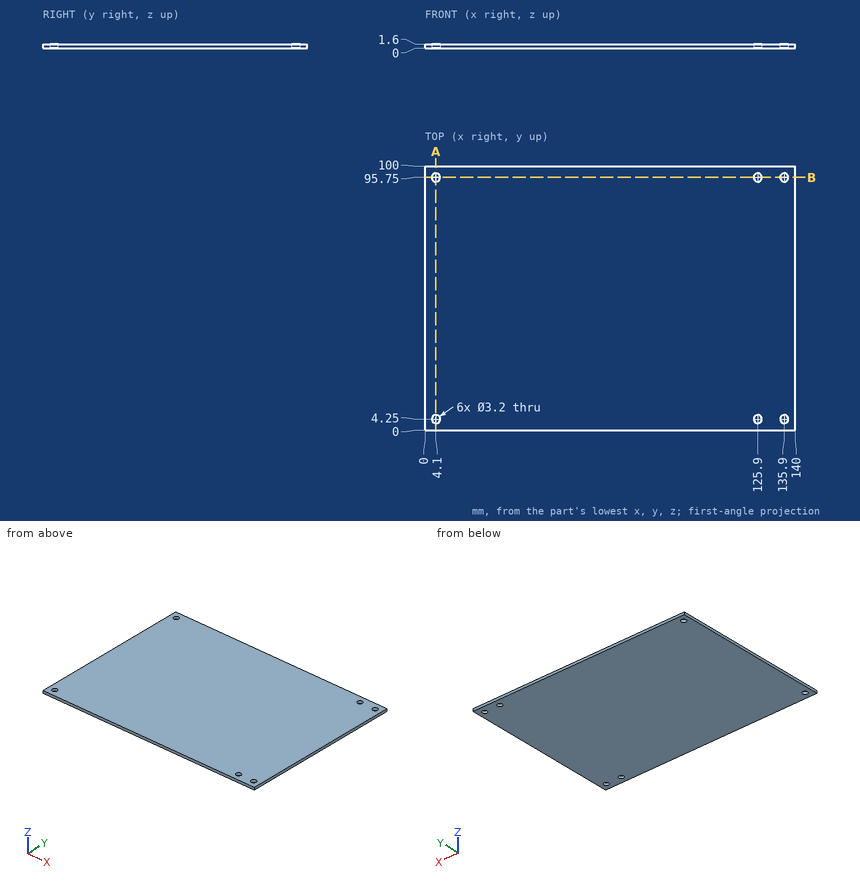
Could you check a few things on this drawing? It's one solid part, dimensions in mm from its lowest x, y, z. Give positions to 0.01 mm unless a question says otherwise; leave off trailing zeros. Write each loop counter-clockwise with the first axis right and the second up, starting at its lowest first coordinate (ties: lowest second). Pieces come first, ordered by that corner, then holes. Notation, with made-up numbers: M 50,-28 L 59,-28 A26 cw 59,-4 Z; hole C -35,12.5 d7. An arc over 180 degrees is marked long. Put each result on its own line as item: value. Start each with the question number.
Item 1: I need wall thicknesses on L1, parallel to X at y = 95.75, z = 0.65; L2, parallel to Y at x = 135.9, z = 0.6. Which ranges of each line are inside material? Lowest first, please. Write a range as from..to.
Item 2: If we section it at B-B, the plane y = 95.75: Write out the boundary of the cut face in (x, z), then the cut area to 3 significant figures.
Item 3: If we section it at A-A, the plane x = 4.1: Write out the boundary of the cut face in (y, z).
Values:
1. L1: 0..2.5, 5.7..124.3, 127.5..134.3, 137.5..140
1. L2: 0..2.65, 5.85..94.15, 97.35..100
2. outline: M 0,0 L 2.5,0 L 2.5,1.6 L 0,1.6 Z; M 5.7,0 L 124.3,0 L 124.3,1.6 L 5.7,1.6 Z; M 127.5,0 L 134.3,0 L 134.3,1.6 L 127.5,1.6 Z; M 137.5,0 L 140,0 L 140,1.6 L 137.5,1.6 Z
2. area: 209 mm²
3. outline: M 0,0 L 2.65,0 L 2.65,1.6 L 0,1.6 Z; M 5.85,0 L 94.15,0 L 94.15,1.6 L 5.85,1.6 Z; M 97.35,0 L 100,0 L 100,1.6 L 97.35,1.6 Z
